```python
from build123d import *

# Parameters (mm, degrees)
SKETCH1_R           = 2.5
BOSS_EXTRUDE1_DEPTH = 3
SKETCH2_R           = 1.5
CUT_EXTRUDE1_DEPTH  = 10


with BuildPart() as part:
    # Sketch1 → Boss-Extrude1 (new body)
    with BuildSketch(Plane.XY):
        with BuildLine():
            Line((-93.660254038, 5), (-8.660254038, 5))
            ThreePointArc((-8.660254038, 5), (10, 0), (-8.660254038, -5))
            Line((-8.660254038, -5), (-93.660254038, -5))
            Line((-93.660254038, -5), (-93.660254038, 5))
        make_face()
        Circle(SKETCH1_R, mode=Mode.SUBTRACT)
    extrude(amount=BOSS_EXTRUDE1_DEPTH)

    # Sketch2 → Cut-Extrude1 (cut)
    with BuildSketch(Plane(origin=(0, 0, 0), x_dir=(-1, 0, 0), z_dir=(0, 0, -1))):
        with Locations((25, 0)):
            Circle(SKETCH2_R)
    extrude(amount=-CUT_EXTRUDE1_DEPTH, mode=Mode.SUBTRACT)


solid = part.part
```
Geometry check sheet. Reference: the model listing, model coordinates, mm. A direction names the side the tool comes from. Coordinates: 2 decimals unless noted, no trailing zeros. Write each loop counter-clockwise with the first axis right and the second up, starting at its lowest first coordinate (ties: lowest second). Pieces come first, ordered by that corner, then holes. Notation, with made-up numbers: M 26,-5 L 69,-5 A27 ccw 69,18 Z; hole C 44.25,-13 d9. An arc over 180 degrees is marked long. Use one line per item in the form item = value. Start each with the question number.
1) Thickness scan on probe 1 along Y at (x, z) = (-25, 1.5); probe 2 along Y at (x, z) = (0, 2.1); probe 3 along Y at (x, z) = (-35, 2.4). Record the ranges inside material, lowest first. Write a range as from..to.
2) Section check A-A on x = -25. Enter the section's corners in (y, z), and give its area (3 significant figures).
3) Set-up check for faces 5 (the flat face through (-52, 5, 1)), 6 (the flat face through (-51, -5, 1)), 7 (the cylindrical face through (-23.5, 0.07, 1.48)): record each of +Z, -Z, +X, -X, +Y, -Y from which the full face is reachable in a straight line by a thin tool's end or side.
4) Section check B-B on y = 0. Enter the section's corners in (x, z).
5) Release check for a two-part mould opening along X. For faces 1 (the cylindrical face through (10, 0, 1)), 2 (the flat face through (-41, 0, 0)), 3 (the cylindrical face through (-0.54, -2.44, 1.48)), 4 (the flat face through (-93.66, 0, 1)) record: pulls with the +X half, pulls with the -X half, needs draft (parallel to the pull), parting line crosses it, or undercut.
6) Section check C-C on z = 1.05. Enter the section's corners in (x, y).
7) Section check D-D on x = 0. Enter the section's corners in (y, z).
8) Go/stop test with flat-tipped pins: pin 1 Ø1 at (x, z) = (-42, 1) entering from -Y; pin 2 Ø2.5 at (x, y) = (-25, 0) entering from +Z. Record where each tip stops, or that it passes through.
Responses:
q1.probe_1 = -5..-1.5, 1.5..5
q1.probe_2 = -10..-2.5, 2.5..10
q1.probe_3 = -5..5
q2.outline = M -5,0 L -1.5,0 L -1.5,3 L -5,3 Z; M 1.5,0 L 5,0 L 5,3 L 1.5,3 Z
q2.area = 21.0 mm2
q3.face_5 = +Z, -Z, -X, +Y
q3.face_6 = +Z, -Z, -X, -Y
q3.face_7 = +Z, -Z
q4.outline = M -93.66,0 L -26.5,0 L -26.5,3 L -93.66,3 Z; M -23.5,0 L -2.5,0 L -2.5,3 L -23.5,3 Z; M 2.5,0 L 10,0 L 10,3 L 2.5,3 Z
q5.face_1 = parting line crosses it
q5.face_2 = needs draft
q5.face_3 = undercut
q5.face_4 = pulls with the -X half
q6.outline = M -93.66,-5 L -8.66,-5 A10 ccw long -8.66,5 L -93.66,5 Z; hole C -25,0 d3; hole C 0,0 d5
q7.outline = M -10,0 L -2.5,0 L -2.5,3 L -10,3 Z; M 2.5,0 L 10,0 L 10,3 L 2.5,3 Z
q8.pin_1 = -5
q8.pin_2 = through
